Can you work these out from the model? Positions are in its coordinate system, mm. A direction names the side the tool comes from. Give positions to 0.01 mm unless a question says otherwise; leave off trailing zeros. Loops run counter-clockwise (first coordinate to the right, second up) from the corner with the lowest first, then second, coordinate; pieces in that order, holes last. Notation, with made-up numbers: M 77,54.5 L 85,54.5 A17 ccw 85,63.5 Z; hole C 85,67.25 d4. An arc over 180 degrees is marked long. Answer as a JSON object with one key per item and string values.
```python
from build123d import *

# Parameters (mm, degrees)
F1_W     = 2.55
F1_H     = 4.1
F1_W_2   = 1.55
F1_H_2   = 3.1
F1_R     = 9.525
F5_DEPTH = 6.35
F3_R     = 9.525
F3_W     = 2.55
F3_H     = 4.1
F6_DEPTH = 6.35


with BuildPart() as f4:
    # F4: sweep along a path in F0
    with BuildLine(Plane.XY) as f4_path:
        Line((0, 0), (0, 10))
        ThreePointArc((0, 10), (-4.510556, 20.889444), (-15.4, 25.4))
        Line((-15.4, 25.4), (-21.85, 25.4))
        Line((-21.85, 25.4), (-28.3, 25.4))
        ThreePointArc((-28.3, 25.4), (-39.189444, 29.910556), (-43.7, 40.8))
        Line((-43.7, 40.8), (-43.7, 50.8))
    # F1 (on Front) → F4 (sweep)
    with BuildSketch(Plane.XZ):
        Rectangle(F1_W, F1_H)
        Rectangle(F1_W_2, F1_H_2, mode=Mode.SUBTRACT)
    sweep(path=f4_path.line)

    # F1 (on Front) → F5 (join)
    with BuildSketch(Plane.XZ):
        Circle(F1_R)
        Rectangle(F1_W, F1_H, mode=Mode.SUBTRACT)
    extrude(amount=-F5_DEPTH)

    # F3 (on offset) → F6 (join)
    with BuildSketch(Plane.XZ.offset(-50.8)):
        with Locations((-43.7, 0)):
            Circle(F3_R)
        with Locations((-43.7, 0)):
            Rectangle(F3_W, F3_H, mode=Mode.SUBTRACT)
    extrude(amount=F6_DEPTH)


solid = f4.part
```
1) For faces 1 (the flat face through (-22, 24.625, 0)), 2 (the flat face through (-44.475, 46, 0)), 3 (the flat face through (-1.275, 8, 0)), which set-ups out of +Z, -Z, +X, -X, +Y, -Y let a thin tool reach every point of the face, with its end or its side?
Answer list:
{"face 1": "none", "face 2": "+Y", "face 3": "+Z, -Z, -X"}
2) Suppose I cut it at A-A, the plane x = -23. Write out the boundary of the cut face in (y, z) (3 decimals), and give its area (3 significant figures).
Answer list:
{"outline": "M 24.125,-2.05 L 26.675,-2.05 L 26.675,2.05 L 24.125,2.05 Z; hole M 24.625,-1.55 L 26.175,-1.55 L 26.175,1.55 L 24.625,1.55 Z", "area": "5.65 mm^2"}
3) Will these pins go through, and if not, where does the flat tip stop? pin 1 Ø22.5 at (x, y) = (-28.5, 24) entering from -Z; pin 2 Ø1.8 at (y, z) = (43, 0.5) entering from +X (3 decimals); pin 3 Ø1.2 at (x, z) = (-25, -0.5) entering from -Y (3 decimals).
Answer list:
{"pin 1": "z = -2.05", "pin 2": "x = -42.425", "pin 3": "y = 24.125"}
4) If we mould it in two halves opening along Y, with no side actions, what happens to faces 4 (the flat face through (-44, 50.8, -2)), 5 (the cylindrical face through (-38.177, 30.703, 0.029)), 6 (the cylindrical face through (-7.559, 3.131, -5.796))? For each: +Y half, -Y half, draft (parallel to the pull), parting line (faces both ways), or undercut.
Answer list:
{"face 4": "+Y half", "face 5": "undercut", "face 6": "draft"}
5) Please list where these lines run through material, in increasing order: line 1 along X through (y, z) = (4.5, 0.25) (3 decimals); line 2 along Z through (x, y) = (-11, 25); line 3 along Y through (x, z) = (-26, 1.25) (3 decimals). Write a range as from..to.
Answer list:
{"line 1": "-9.522..-0.775, 0.775..9.522", "line 2": "-2.05..-1.55, 1.55..2.05", "line 3": "24.125..24.625, 26.175..26.675"}
6) Suppose I cut it at C-C, the plane x = -3. Write out the boundary of the cut face in (y, z).
Answer list:
{"outline": "M 0,-9.04 L 6.35,-9.04 L 6.35,9.04 L 0,9.04 Z; M 16.76,-2.05 L 21.15,-2.05 L 21.15,2.05 L 16.76,2.05 Z; hole M 17.75,-1.55 L 20.39,-1.55 L 20.39,1.55 L 17.75,1.55 Z"}
7) Suppose I cut it at D-D, the plane y = 28.5. Write out the boundary of the cut face in (x, z).
Answer list:
{"outline": "M -39.56,-2.05 L -35.24,-2.05 L -35.24,2.05 L -39.56,2.05 Z; hole M -38.8,-1.55 L -36.21,-1.55 L -36.21,1.55 L -38.8,1.55 Z"}
